Can you work these out from the model? Positions are in its coordinate system, mm. A direction names the side the tool comes from. Round coordinates to 2 decimals unless told otherwise and drop trailing zeros. Write each loop counter-clockwise with the first axis right and the second up, starting at its lowest first coordinate (ties: lowest second). Pieces come first, ordered by that corner, then holes. Notation, with made-up numbers: M -18.75,63 L 5.25,63 A20 ccw 5.25,89 Z; hole C 86,87.25 d4. An arc over 180 degrees is marked long. Answer as a JSON object with one key per item and string values. Group by question number.
1) If we mould it in two halves opening along Y, with no side actions, what happens to faces 3 (the cylindrical face through (30.04, 87.54, 95.38)), 4 (the flat face through (-43, 85, -1)), 5 (the flat face through (24, 0, 21))? For each: +Y half, -Y half, draft (parallel to the pull), parting line (faces both ways), or undercut.
2) Suppose I cut it at D-D, the plane x = 53. Write out the boundary of the cut face in (y, z).
3) I'm going to push flat-ended pins straight in: pin 1 Ø1 at (y, z) = (40.5, -36) entering from -X; pin 2 Ø5 at (x, y) = (32, 66.5) entering from -Z; pin 3 Ø5 at (y, z) = (15.5, -30) entering from +X; pin 4 Ø3 at (y, z) = (47, -3) entering from -X. Where does each tip first touch, or does it pass through?
4) Suppose I cut it at C-C, the plane y = 40. Write out the boundary of the cut face in (x, z).
5) Please list where these lines run through material, in increasing order: L1, parallel to Z at x = -1, y = 60.5; L2, parallel to Y at x = 62, z = -4.5; L3, parallel to X at y = 87, z = 0. Write a range as [from, to].
6) On a 3-axis mill with a long thin cutter (end or side, diameter ignored), from which of +Z, -Z, +X, -X, +Y, -Y can I reach the whole of each face in a straight line? I mean faces 1 (the cylindrical face through (30.04, 2.46, 95.38)), 2 (the flat face through (-43, 5, -1)). Say none if no direction works.
7) Suppose I cut it at A-A, the plane x = 0. Write out the boundary of the cut face in (y, z), and give its area (3 significant figures).
8) Suppose I cut it at B-B, the plane z = 0. Write out the boundary of the cut face in (x, y), and give its area (3 significant figures).
from build123d import *

# Parameters (mm, degrees)
SKETCH1_R           = 100
SKETCH1_R_2         = 30
BOSS_EXTRUDE1_DEPTH = 5
SKETCH2_R           = 35
SKETCH2_R_2         = 30
BOSS_EXTRUDE2_DEPTH = 40


with BuildPart() as part:
    # Sketch1 → Boss-Extrude1 (new body)
    with BuildSketch(Plane(origin=(0, 0, 0), x_dir=(1, 0, 0), z_dir=(0, 1, 0))):
        with Locations(Location((0, 0, 0), (0, 0, 270))):
            Circle(SKETCH1_R)
        with Locations(Location((0, 0, 0), (0, 0, 270))):
            Circle(SKETCH1_R_2, mode=Mode.SUBTRACT)
    boss_extrude1 = extrude(amount=BOSS_EXTRUDE1_DEPTH)

    # Sketch2 → Boss-Extrude2 (add)
    with BuildSketch(Plane(origin=(0, 5, 0), x_dir=(1, 0, 0), z_dir=(0, 1, 0))):
        with Locations(Location((0, 0, 0), (0, 0, 270))):
            Circle(SKETCH2_R)
        with Locations(Location((0, 0, 0), (0, 0, 270))):
            Circle(SKETCH2_R_2, mode=Mode.SUBTRACT)
    boss_extrude2 = extrude(amount=BOSS_EXTRUDE2_DEPTH)

    # Mirror1: Boss-Extrude1, Boss-Extrude2 across plane
    add(boss_extrude1.mirror(Plane.ZX.offset(45)))
    add(boss_extrude2.mirror(Plane.ZX.offset(45)))


solid = part.part
Results:
{
 "1": {"face 3": "draft", "face 4": "undercut", "face 5": "-Y half"},
 "2": {"outline": "M 0,-84.8 L 5,-84.8 L 5,84.8 L 0,84.8 Z; M 85,-84.8 L 90,-84.8 L 90,84.8 L 85,84.8 Z"},
 "3": {"pin 1": "through", "pin 2": "z = -18.83", "pin 3": "x = 21.65", "pin 4": "x = -34.97"},
 "4": {"outline": "C 0,0 d70; hole C 0,0 d60"},
 "5": {"L1": "[-34.99, -29.98], [29.98, 34.99]", "L2": "[0, 5], [85, 90]", "L3": "[-100, -30], [30, 100]"},
 "6": {"face 1": "+Y, -Y", "face 2": "none"},
 "7": {"outline": "M 0,-100 L 5,-100 L 5,-35 L 85,-35 L 85,-100 L 90,-100 L 90,-30 L 0,-30 Z; M 0,30 L 90,30 L 90,100 L 85,100 L 85,35 L 5,35 L 5,100 L 0,100 Z", "area": "2,200 mm^2"},
 "8": {"outline": "M -100,0 L -30,0 L -30,90 L -100,90 L -100,85 L -35,85 L -35,5 L -100,5 Z; M 30,0 L 100,0 L 100,5 L 35,5 L 35,85 L 100,85 L 100,90 L 30,90 Z", "area": "2,200 mm^2"}
}
